```python
from build123d import *

# Parameters (mm, degrees)
F0_R     = 39.7343740688
F1_DEPTH = 75.946
F3_DEPTH = 29.21
F3_TAPER = 45


with BuildPart() as f1:
    # F0 (on Top) → F1 (new body)
    with BuildSketch(Plane.XY):
        Circle(F0_R)
    extrude(amount=F1_DEPTH)

    # F2 (on face) → F3 (cut)
    with BuildSketch(Plane.XY.offset(75.946)):
        Polygon((37.6749132279, 0.2816330117), (18.5935552713, 32.7682484466), (-19.0813579566, 32.4866154349), (-37.6749132279, -0.2816330117), (-18.5935552713, -32.7682484466), (19.0813579566, -32.4866154349), align=None)
    extrude(amount=-F3_DEPTH, taper=F3_TAPER, mode=Mode.SUBTRACT)


solid = f1.part
```
Geometry check sheet. Reference: the model listing, model coordinates, mm. Round coordinates to 2 decimals unless told otherwise and drop trailing zeros. Loops run counter-clockwise (first coordinate to the right, second up) from the corner with the lowest first, then second, coordinate; pieces in that order, holes last. Notation, with made-up numbers: M 55.25,-22 L 72.25,-22 A18 cw 72.25,-6 Z; hole C -38,17.25 d7. An arc over 180 degrees is marked long. Return JSON: item names as keys, results as strings. Group by question number.
(1) Mould release check, pull along Y, two halves, no side actions. Record for faces 1 (the face through (0, 0, 46.736)), 2 (the face through (-8.61, -38.79, 37.44)), 3 (the face through (-30, -15, 75.946)): pulls with the +Y half, pulls with the -Y half, needs draft (parallel to the pull), parting line crosses it, or undercut.
(2) Section check A-A, the plane z = 15. Enter the section's corners in (x, y).
(3) Scan lines: line 1 along Y through (x, z) = (4, 71); line 2 along X through (y, z) = (-22.5, 37); line 3 along Y through (x, z) = (14.5, 72). Record each from-to range of solid material in increasing order. Write a range as [from, to].
(4) Go/stop test with flat-tipped pins: pin 1 (8 mm diameter, centred on x = -31, y = -23.5, fed in from -Z); pin 2 (6 mm diameter, centred on x = -14.5, z = 21, fed in from -Y); pin 3 (3 mm diameter, centred on x = -27.5, z = 48, fed in from -Y); pin 4 (4 mm diameter, centred on x = 31, z = 55.5, fed in from -Y). Record where each tip stops, or that it passes through.
Data:
{
 "1": {"face 1": "undercut", "face 2": "parting line crosses it", "face 3": "needs draft"},
 "2": {"outline": "C 0,0 d79.47"},
 "3": {"line 1": "[-39.53, -27.65], [27.71, 39.53]", "line 2": "[-32.75, 32.75]", "line 3": "[-36.99, -28.57], [28.79, 36.99]"},
 "4": {"pin 1": "z = 0", "pin 2": "y = -38.03", "pin 3": "y = -30.05", "pin 4": "y = -27.16"}
}
